Part print with two shaded views. Sizes in mm from the minimum x, y, z corner. Round coordinates to 2 decimals unless told otherwise and drop trailing zeros. Write each loop counter-clockwise with the first axis right and the second up, starting at its lowest first coordinate (ties: lowest second). Pieces come first, ordered by that corner, then holes. Notation, with made-up numbers: (-9.75, 33) -> (-0.75, 33) arc R24 ccw to (-0.75, 49) -> close; hole circle Ø9 at (-4.5, 87.25). An arc over 180 degrees is marked (long way). Put each result on its own line as item: value. Start each with the question number.
1. Saw through at D-D on y = 11.75. List the corners of the cut face in (x, z), and give its area (3 significant figures).
2. Drill centre lines: line 1 (X direction, y = 4.75, z = 17) (1 decimal); line 2 (Y direction, x = 4.75, z = 16.5) (1 decimal); line 3 (Y direction, x = 5, z = 15.25). Where is each one in solid material? Low to high. Write a range as from..to.
3. Saw through at C-C on y = 6. List the corners of the cut face in (x, z).
4. Saw through at A-A on x = 10.5. List the corners of the cut face in (y, z), and give its area (3 significant figures).
5. Flat gauge pin, fed straight in: P1, Ø1.2, axis at y = 11, z = 8, coming from the +X side. Where does the tip first touch, or does it go through?
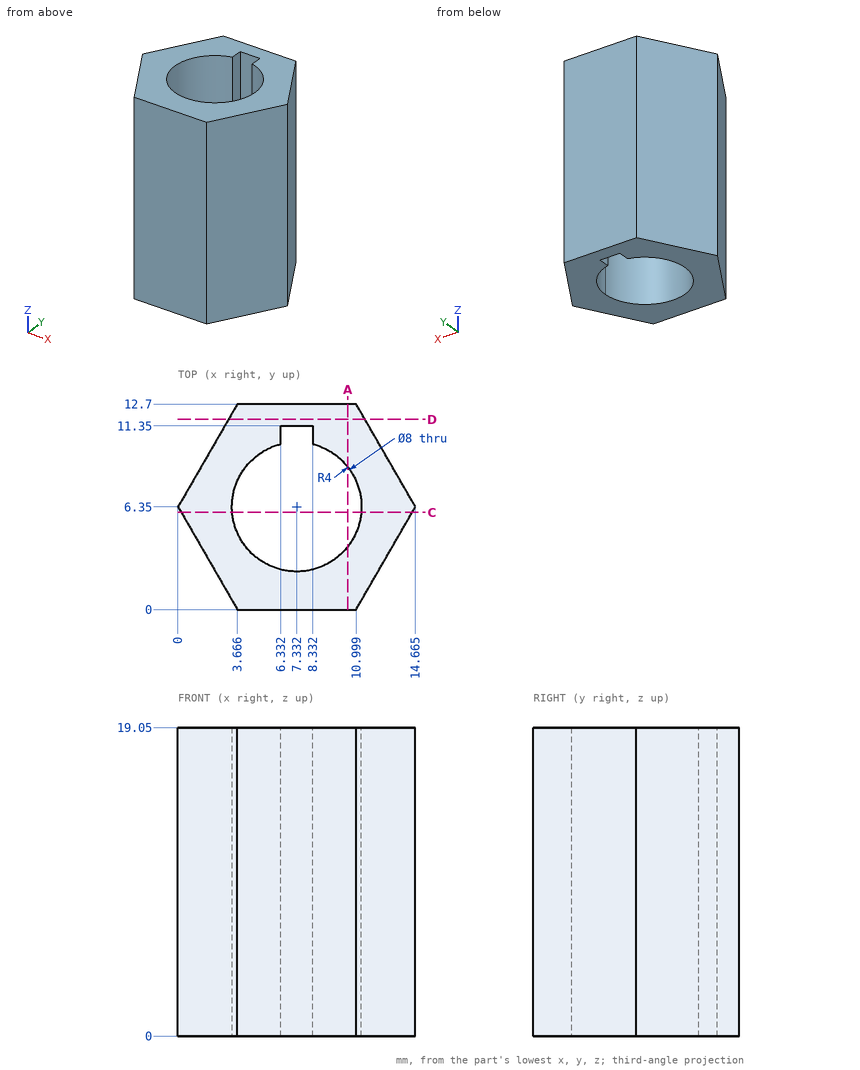
Return value:
1. outline: (3.12, 0) -> (11.55, 0) -> (11.55, 19.05) -> (3.12, 19.05) -> close
1. area: 161 mm^2
2. line 1: x = 0.9..3.7, 11..13.7
2. line 2: y = 0..3.3, 9.4..12.7
2. line 3: y = 0..3.1, 9.6..12.7
3. outline: (0.2, 0) -> (3.35, 0) -> (3.35, 19.05) -> (0.2, 19.05) -> close; (11.32, 0) -> (14.46, 0) -> (14.46, 19.05) -> (11.32, 19.05) -> close
4. outline: (0, 0) -> (3.91, 0) -> (3.91, 19.05) -> (0, 19.05) -> close; (8.79, 0) -> (12.7, 0) -> (12.7, 19.05) -> (8.79, 19.05) -> close
4. area: 149 mm^2
5. P1: stops at x = 12.33
